from build123d import *

# Parameters (mm, degrees)
F1_DEPTH = 12.7
F2_SIZE  = 3.17499
F3_SIZE  = 3.17499


# Not quite as in the source:
# - a fillet or chamfer is up to 0.001 mm smaller than in the source, because OpenCascade refuses the exact size


with BuildPart() as f1:
    # F0 (on Top) → F1 (new body)
    with BuildSketch(Plane.XY):
        Polygon((42.3333333333, 73.3234841871), (0, 146.6469683742), (-42.3333333333, 73.3234841871), (-127, 73.3234841871), (-84.6666666667, 0), (-127, -73.3234841871), (-42.3333333333, -73.3234841871), (0, -146.6469683742), (42.3333333333, -73.3234841871), (127, -73.3234841871), (84.6666666667, 0), (127, 73.3234841871), align=None)
        with BuildLine():
            ThreePointArc((107.7525859006, 66.9734850526), (111.8770318861, 64.5922350526), (111.8770318861, 59.8297350526))
            Line((111.8770318861, 59.8297350526), (42.3333325205, -60.623485595))
            Line((42.3333325205, -60.623485595), (49.6656809392, -60.623485595))
            Line((49.6656809392, -60.623485595), (76.8760464718, -13.49375))
            ThreePointArc((76.8760464718, -13.49375), (81.0004924573, -11.1125), (85.1249384428, -13.49375))
            Line((85.1249384428, -13.49375), (111.8770318861, -59.8297350526))
            ThreePointArc((111.8770318861, -59.8297350526), (111.8770318861, -64.5922350526), (107.7525859006, -66.9734850526))
            Line((107.7525859006, -66.9734850526), (-31.3348102056, -66.9734850526))
            Line((-31.3348102056, -66.9734850526), (-27.6686364959, -73.3234841871))
            Line((-27.6686364959, -73.3234841871), (26.7520929436, -73.3234841871))
            ThreePointArc((26.7520929436, -73.3234841871), (30.8765389291, -75.7047341871), (30.8765389291, -80.4672341871))
            Line((30.8765389291, -80.4672341871), (4.1244459855, -126.8032183742))
            ThreePointArc((4.1244459855, -126.8032183742), (0, -129.1844683742), (-4.1244459855, -126.8032183742))
            Line((-4.1244459855, -126.8032183742), (-73.6681446525, -6.3499989368))
            Line((-73.6681446525, -6.3499989368), (-77.3343188618, -12.6999989368))
            Line((-77.3343188618, -12.6999989368), (-50.1239530285, -59.8297350526))
            ThreePointArc((-50.1239530285, -59.8297350526), (-50.1239530285, -64.5922350526), (-54.2483990141, -66.9734850526))
            Line((-54.2483990141, -66.9734850526), (-107.7525871283, -66.9734850526))
            ThreePointArc((-107.7525871283, -66.9734850526), (-111.8770331138, -64.5922350526), (-111.8770331138, -59.8297350526))
            Line((-111.8770331138, -59.8297350526), (-42.3333337482, 60.623485595))
            Line((-42.3333337482, 60.623485595), (-49.6656809392, 60.623485595))
            Line((-49.6656809392, 60.623485595), (-76.8760464718, 13.49375))
            ThreePointArc((-76.8760464718, 13.49375), (-81.0004924573, 11.1125), (-85.1249384428, 13.49375))
            Line((-85.1249384428, 13.49375), (-111.8770318861, 59.8297350526))
            ThreePointArc((-111.8770318861, 59.8297350526), (-111.8770318861, 64.5922350526), (-107.7525859006, 66.9734850526))
            Line((-107.7525859006, 66.9734850526), (31.3348102056, 66.9734850526))
            Line((31.3348102056, 66.9734850526), (27.6686364959, 73.3234841871))
            Line((27.6686364959, 73.3234841871), (-26.7520941713, 73.3234841871))
            ThreePointArc((-26.7520941713, 73.3234841871), (-30.8765401568, 75.7047341871), (-30.8765401568, 80.4672341871))
            Line((-30.8765401568, 80.4672341871), (-4.1244465994, 126.8032194374))
            ThreePointArc((-4.1244465994, 126.8032194374), (-6.138e-07, 129.1844694374), (4.1244453717, 126.8032194374))
            Line((4.1244453717, 126.8032194374), (73.6681440386, 6.35))
            Line((73.6681440386, 6.35), (77.334318248, 12.7))
            Line((77.334318248, 12.7), (50.1239530285, 59.8297350526))
            ThreePointArc((50.1239530285, 59.8297350526), (50.1239530285, 64.5922350526), (54.248399014, 66.9734850526))
            Line((54.248399014, 66.9734850526), (107.7525859006, 66.9734850526))
        make_face(mode=Mode.SUBTRACT)
    extrude(amount=F1_DEPTH)

    # F2 (size 3.175 in the source; OpenCascade refuses exactly that, so slightly less here)
    f2_edges = [f1.edges().sort_by_distance(p)[0] for p in [
        (105.833333, -36.661742, 12.7),
        (105.833333, 36.661742, 12.7),
        (84.666667, 73.323484, 12.7),
        (21.166667, 109.985226, 12.7),
        (-21.166667, 109.985226, 12.7),
        (-84.666667, 73.323484, 12.7),
        (-105.833333, 36.661742, 12.7),
        (-105.833333, -36.661742, 12.7),
        (-84.666667, -73.323484, 12.7),
        (-21.166667, -109.985226, 12.7),
        (21.166667, -109.985226, 12.7),
        (84.666667, -73.323484, 12.7),
        (38.896295, 66.57661, 12.7),
        (75.501231, 9.525, 12.7),
        (63.729136, 36.264868, 12.7),
        (50.123953, 64.592235, 12.7),
        (81.000492, 66.973485, 12.7),
        (111.877032, 64.592235, 12.7),
        (77.105182, -0.396875, 12.7),
        (45.999507, -60.623486, 12.7),
        (63.270864, -37.058618, 12.7),
        (81.000492, -11.1125, 12.7),
        (98.500985, -36.661743, 12.7),
        (111.877032, -64.592235, 12.7),
        (38.208888, -66.973485, 12.7),
        (-29.501723, -70.148485, 12.7),
        (-0.458272, -73.323484, 12.7),
        (30.876539, -75.704734, 12.7),
        (17.500492, -103.635226, 12.7),
        (0, -129.184468, 12.7),
        (-38.896295, -66.576609, 12.7),
        (-75.501232, -9.524999, 12.7),
        (-63.729136, -36.264867, 12.7),
        (-50.123953, -64.592235, 12.7),
        (-81.000493, -66.973485, 12.7),
        (-111.877033, -64.592235, 12.7),
        (-77.105183, 0.396875, 12.7),
        (-45.999507, 60.623486, 12.7),
        (-63.270864, 37.058618, 12.7),
        (-81.000492, 11.1125, 12.7),
        (-98.500985, 36.661743, 12.7),
        (-111.877032, 64.592235, 12.7),
        (-38.208888, 66.973485, 12.7),
        (29.501723, 70.148485, 12.7),
        (0.458271, 73.323484, 12.7),
        (-30.87654, 75.704734, 12.7),
        (-17.500493, 103.635227, 12.7),
        (-1e-06, 129.184469, 12.7),
    ]]
    chamfer(f2_edges, length=F2_SIZE)

    # F3 (size 3.175 in the source; OpenCascade refuses exactly that, so slightly less here)
    f3_edges = [f1.edges().sort_by_distance(p)[0] for p in [
        (105.833333, -36.661742, 0),
        (105.833333, 36.661742, 0),
        (84.666667, 73.323484, 0),
        (21.166667, 109.985226, 0),
        (-21.166667, 109.985226, 0),
        (-84.666667, 73.323484, 0),
        (-105.833333, 36.661742, 0),
        (-105.833333, -36.661742, 0),
        (-84.666667, -73.323484, 0),
        (-21.166667, -109.985226, 0),
        (21.166667, -109.985226, 0),
        (84.666667, -73.323484, 0),
        (38.896295, 66.57661, 0),
        (75.501231, 9.525, 0),
        (63.729136, 36.264868, 0),
        (50.123953, 64.592235, 0),
        (81.000492, 66.973485, 0),
        (111.877032, 64.592235, 0),
        (77.105182, -0.396875, 0),
        (45.999507, -60.623486, 0),
        (63.270864, -37.058618, 0),
        (81.000492, -11.1125, 0),
        (98.500985, -36.661743, 0),
        (111.877032, -64.592235, 0),
        (38.208888, -66.973485, 0),
        (-29.501723, -70.148485, 0),
        (-0.458272, -73.323484, 0),
        (30.876539, -75.704734, 0),
        (17.500492, -103.635226, 0),
        (0, -129.184468, 0),
        (-38.896295, -66.576609, 0),
        (-75.501232, -9.524999, 0),
        (-63.729136, -36.264867, 0),
        (-50.123953, -64.592235, 0),
        (-81.000493, -66.973485, 0),
        (-111.877033, -64.592235, 0),
        (-77.105183, 0.396875, 0),
        (-45.999507, 60.623486, 0),
        (-63.270864, 37.058618, 0),
        (-81.000492, 11.1125, 0),
        (-98.500985, 36.661743, 0),
        (-111.877032, 64.592235, 0),
        (-38.208888, 66.973485, 0),
        (29.501723, 70.148485, 0),
        (0.458271, 73.323484, 0),
        (-30.87654, 75.704734, 0),
        (-17.500493, 103.635227, 0),
        (-1e-06, 129.184469, 0),
    ]]
    chamfer(f3_edges, length=F3_SIZE)


solid = f1.part
Can you work these out from the model? Positions are in its coordinate system, mm. A direction names the side the tool comes from. Give positions to 0.01 mm unless a question says otherwise; leave off trailing zeros. One line per item, written item: value.
1) Thinking about a two-plate mould opening in Y: for faces 1 (the face through (-20.572, -107.884, 1.61)), 2 (the face through (-75.476, -9.481, 6.306)), 3 (the face through (20.534, 107.862, 11.135)), which applies, +Y half, -Y half, draft (parallel to the pull), parting line (faces both ways), or undercut?
Geometry check:
face 1: -Y half
face 2: undercut
face 3: +Y half
2) Please list where these lines run through material, in increasing order: line 1 (X direction, y = -24.5, z = 4.5); line 2 (Y direction, x = 67.5, z = 11); line 3 (X direction, y = 66, z = 8.75).
Geometry check:
line 1: x = -98.81 to -91.48, -70.52 to -63.19, 63.19 to 70.52, 91.48 to 98.81
line 2: y = -71.85 to -68.45, -26.78 to -19.98, 19.98 to 26.78, 68.45 to 71.85
line 3: x = -122.77 to -110.64, 39.23 to 51.36, 110.64 to 122.77
3) I'm going to push flat-ended pins straight in: pin 1 (3 mm diameter, centred on x = 73.5, z = 7.5, fed in from +Y); pin 2 (12 mm diameter, centred on x = -42.5, y = 79.5, fed in from +Z); pin 3 (3 mm diameter, centred on x = -91, z = 7, fed in from -Y). Where does each tip first touch, or does it pass through?
Geometry check:
pin 1: stops at y = 73.32
pin 2: stops at z = 12.29
pin 3: stops at y = -73.32
4) Imagine slicing it at A-A on y = -47. Count the separate pieces of the cut face and the enclosed holes in it, and give its area (3 significant figures).
Geometry check:
separate pieces: 4
enclosed holes: 0
area: 279 mm²
5) On a 3-axis mill with a long thin cutter (end or side, diameter ignored), from which of +Z, -Z, +X, -X, +Y, -Y can I reach the whole of each face in a straight line? I mean faces 4 (the face through (-19.082, 104.116, 11.135)), 5 (the face through (19.043, -104.094, 1.61)), 6 (the face through (-0.07, 129.184, 6.306)). Say none if no direction works.
Geometry check:
face 4: +Z
face 5: -Z
face 6: +Z, -Z
